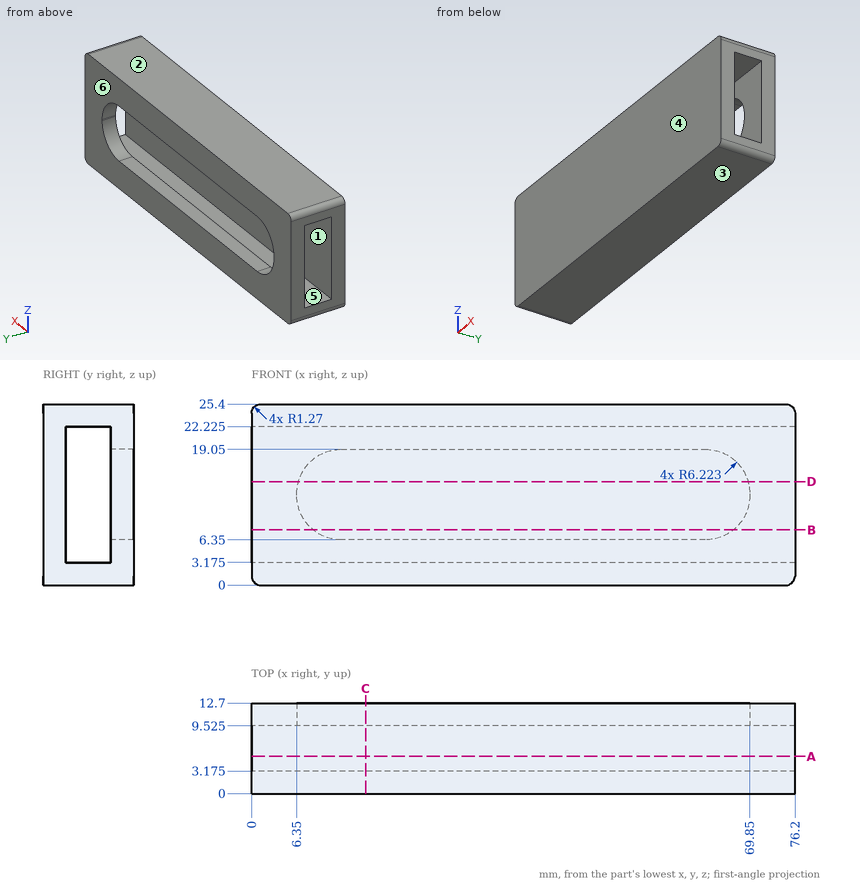
Answer from the drawing. Dimensions are ordinates in mm from the lowest x, y and z of the part. A direction names the side the tool comes from. Give positions to 0.01 mm unless a question says otherwise; leave off trailing zeros. Order: outer loops, then holes, each group sorted by start corner. A loop starts at its lowest first (then second) coordinate and runs counter-clockwise, first axis right, second up. Notation, with made-up numbers: (46, -35.75) - (80, -35.75) arc R21 ccw to (80, -22.75) - close; hole circle Ø7 at (76, 58). An arc over 180 degrees is marked (long way). One line per item, written item: value. Start each with the question number.
1) The mould has two halves that part along Y. Classify the marked faces 3, 4, 5 and 6: released by +Y, released by -Y, zero draft, split by the parting line, or undercut.
2) Find the intervals of material crossed by L1, parallel to Z at x = 30.5, y = 11.25; L2, parallel to Z at x = 20, y = 3.5 (3 decimals); L3, parallel to Y at x = 62, z = 21.5 (3 decimals), in increasing order.
3) A tool of negligible diameter and unlimited length cuts with its end or side. For the marked faces 1 and 2, from which of +Z, -Z, +X, -X, +Y, -Y can it reach the whole face along a straight path? Write none if from no direction.
4) A cutting plane is placed at D-D on z = 14.5. Give the vertices of the cut face in (x, y) (3 decimals), then the cut area to 3 significant figures.
5) A cutting plane is placed at A-A on y = 5.25. Give the vertices of the cut face in (x, z) (3 decimals), then the cut area to 3 significant figures.
6) A cutting plane is placed at B-B on z = 7.75. Give the vertices of the cut face in (x, y) (3 decimals).
7) A cutting plane is placed at C-C on x = 16. Give the vertices of the cut face in (y, z) (3 decimals).
Answer sheet:
1. face 3: zero draft
1. face 4: released by -Y
1. face 5: undercut
1. face 6: released by +Y
2. L1: z = 0 to 6.35, 19.05 to 25.4
2. L2: z = 0 to 3.175, 22.225 to 25.4
2. L3: y = 0 to 3.175, 9.525 to 12.7
3. face 1: +X, -X
3. face 2: +Z, +X, -X, +Y, -Y
4. outline: (0, 0) - (76.2, 0) - (76.2, 3.175) - (0, 3.175) - close; (0, 9.525) - (6.579, 9.525) - (6.579, 12.7) - (0, 12.7) - close; (69.621, 9.525) - (76.2, 9.525) - (76.2, 12.7) - (69.621, 12.7) - close
4. area: 284 mm2
5. outline: (0, 1.27) arc R1.27 ccw to (1.27, 0) - (74.93, 0) arc R1.27 ccw to (76.2, 1.27) - (76.2, 3.175) - (0, 3.175) - close; (0, 22.225) - (76.2, 22.225) - (76.2, 24.13) arc R1.27 ccw to (74.93, 25.4) - (1.27, 25.4) arc R1.27 ccw to (0, 24.13) - close
5. area: 482 mm2
6. outline: (0, 0) - (76.2, 0) - (76.2, 3.175) - (0, 3.175) - close; (0, 9.525) - (8.641, 9.525) - (8.641, 12.7) - (0, 12.7) - close; (67.559, 9.525) - (76.2, 9.525) - (76.2, 12.7) - (67.559, 12.7) - close
7. outline: (0, 0) - (12.7, 0) - (12.7, 6.35) - (9.525, 6.35) - (9.525, 3.175) - (3.175, 3.175) - (3.175, 22.225) - (9.525, 22.225) - (9.525, 19.05) - (12.7, 19.05) - (12.7, 25.4) - (0, 25.4) - close
